from build123d import *

# Parameters (mm, degrees)
SKETCH3_W          = 1.3
SKETCH3_H          = 4.4
CUT_EXTRUDE1_DEPTH = 5
CUT_EXTRUDE2_DEPTH = 10


with BuildPart() as part:
    # Sketch2 → Loft1 section 0
    with BuildSketch(Plane.XY.offset(9)):
        with BuildLine():
            Line((-3.5, 8.5), (3.5, 8.5))
            Line((3.5, 8.5), (3.5, -8.5))
            Line((3.5, -8.5), (-3.5, -8.5))
            Line((-3.5, -8.5), (-3.5, 8.5))
        make_face()
    # Sketch1 → Loft1 section 1
    with BuildSketch(Plane.XY):
        with BuildLine():
            Line((-4.5, 11), (4.5, 11))
            Line((4.5, 11), (4.5, -11))
            Line((4.5, -11), (-4.5, -11))
            Line((-4.5, -11), (-4.5, 11))
        make_face()
    loft()

    # Sketch3 → Cut-Extrude1 (cut)
    with BuildSketch(Plane(origin=(0, 0, 0), x_dir=(-1, 0, 0), z_dir=(0, 0, -1))):
        Rectangle(SKETCH3_W, SKETCH3_H)
    extrude(amount=-CUT_EXTRUDE1_DEPTH, mode=Mode.SUBTRACT)

    # Sketch4 → Cut-Extrude2 (cut, symmetric)
    with BuildSketch(Plane(origin=(0, 0, 0), x_dir=(0, 0, -1), z_dir=(1, 0, 0))):
        with BuildLine():
            Line((-9.861070231, 7.982564486), (-10.140578955, -8.37058785))
            ThreePointArc((-10.140578955, -8.37058785), (-7.362485205, -0.239106283), (-9.861070231, 7.982564486))
        make_face()
    extrude(amount=CUT_EXTRUDE2_DEPTH, both=True, mode=Mode.SUBTRACT)


solid = part.part
For this review, take the finished solid that the model builds, in its own axes (mm). A direction names the side the tool comes from. Give positions to 0.01 mm unless a question says otherwise; leave off trailing zeros. Write each question's results on one line, items separated by ' | '.
(1) For line 1 along Z through (x, y) = (0.5, 0.25); line 2 along Y through (x, z) = (0.25, 4.5); line 3 along Y through (x, z) = (0.5, 2.75), list the stretches that pass through material, from the lowest coordinate up.
Conclusion:
line 1: 5 to 7.36 | line 2: -9.75 to -2.2, 2.2 to 9.75 | line 3: -10.24 to -2.2, 2.2 to 10.24
(2) For faces 3 (the flat face through (0, 2.2, 2)), 4 (the flat face through (-2, -1, 0)), list the 3-axis set-ups (+Z, -Z, +X, -X, +Y, -Y) from which the entire face can be reached by the end or side of a thin tool; tool diameter is ignored.
Conclusion:
face 3: -Z | face 4: -Z, +X, -X, +Y, -Y
(3) For pin 1 Ø1.4 at (x, z) = (0, 2.5) entering from -Y; pin 2 Ø4 at (y, z) = (3.5, 6) entering from -X; pin 3 Ø1.4 at (x, z) = (-0.5, 2) entering from +Y, all flat-tipped, find the tip position at first contact; note any pin that passes through.
Conclusion:
pin 1: y = -10.5 | pin 2: x = -4.06 | pin 3: y = 10.64
(4) Draft analysis for pull direction X (two halves, no side actions). For faces 1 (the flat face through (0.65, 0, 2)), 2 (the flat face through (0, -7, 9)), state which applies: +X half, -X half, draft (parallel to the pull), parting line (faces both ways), or undercut.
Conclusion:
face 1: undercut | face 2: draft
